from build123d import *

# Parameters (mm, degrees)
AXLE_BASE_SKETCH_R        = 15.5
AXLE_DEPTH                = 92
GUARD_BASE_R              = 25
GUARD_DEPTH               = 5
INNER_AXLE_HOLE_BASE_R    = 10
INNER_AXLE_HOLE_DEPTH     = 104.242433137
COUPLING_TOOTH_HOLE_DEPTH = 4


with BuildPart() as part:
    # Axle base sketch → Axle (new body)
    with BuildSketch(Plane.XY):
        Circle(AXLE_BASE_SKETCH_R)
    extrude(amount=AXLE_DEPTH)

    # Guard base → Guard (add)
    with BuildSketch(Plane(origin=(0, 0, 0), x_dir=(-1, 0, 0), z_dir=(0, 0, -1))):
        Circle(GUARD_BASE_R)
    extrude(amount=GUARD_DEPTH)

    # Inner axle hole base → Inner axle hole (cut, through all)
    with BuildSketch(Plane.XY.offset(92)):
        Circle(INNER_AXLE_HOLE_BASE_R)
    extrude(amount=-INNER_AXLE_HOLE_DEPTH, mode=Mode.SUBTRACT)

    # Coupling tooth base → Coupling tooth hole (cut, symmetric)
    with BuildSketch(Plane(origin=(0, 0, 0), x_dir=(1, 0, 0), z_dir=(0, 1, 0))):
        Polygon((12.5, -89.5), (10, -92), (15.5, -92), (15.5, -79), (12.5, -79), (11.5, -80), (11.5, -82), (12.5, -83), align=None)
    coupling_tooth_hole = extrude(amount=COUPLING_TOOTH_HOLE_DEPTH, both=True, mode=Mode.SUBTRACT)

    # Coupling teeth: Coupling tooth hole across plane
    add(coupling_tooth_hole.mirror(Plane(origin=(0, 0, 0), x_dir=(0, 0, 1), z_dir=(1, 0, 0))), mode=Mode.SUBTRACT)


solid = part.part
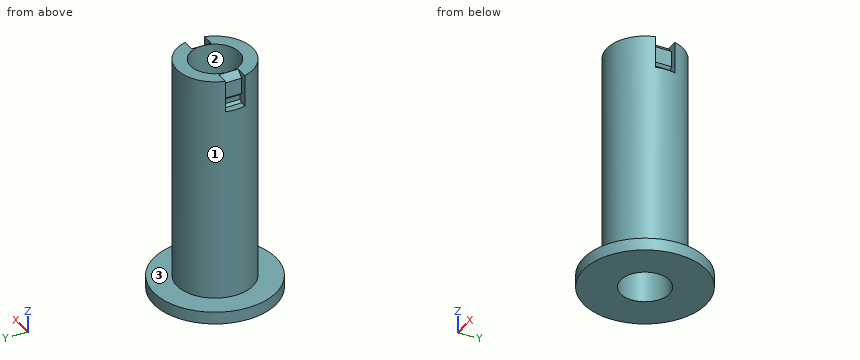
Could you check a few things on this model? Use its own coordinates, in mm. Face numbers are marked on the shaded views. Give positions to 0.01 mm unless a question says otherwise; leave off trailing zeros. Order: outer loops, then holes, each group sorted by start corner. A loop starts at its lowest first (then second) coordinate and runs counter-clockwise, first axis right, second up.
1. Suppose I cut it at D-D (y = -14.5). List the corners of the cut face in (x, z) for me.
2. Will these pins go through, and if not, where does the flat tip stop? P1, Ø12, axis at x = 15.5, z = 22, coming from the +Y side; P2, Ø5, axis at x = -18.5, y = -18.5, coming from the +Z side; P3, Ø12, axis at x = 15, z = 65.5, coming from the -Y side; P4, Ø12, axis at x = -9, y = -18.5, coming from the +Z side.
3. Suppose I cut it at C-C (z = 70.5). List the corners of the cut face in (x, y) for me.
4. Suppose I cut it at B-B (y = -6.5). List the corners of the cut face in (x, z) for me, plus the area to 3 significant figures.
5. I need wall thicknesses on L1, parallel to Y at x = 0, z = 22; L2, parallel to Z at x = -11, y = -15.5; L3, parallel to Y at x = 8.5, z = 10.5. Which ranges of each line are inside material? Lowest first, please.
6. Suppose I cut it at A-A (x = 0). List the corners of the cut face in (y, z) for me, plus the area to 3 significant figures.
7. We'd pull the mould along Y, two halves only. Please class the marked faces 1, 2 and 3: pulls with the +Y half, pulls with the -Y half, needs draft (parallel to the pull), parting line crosses it, or undercut.
Solved:
1. outline: (-20.37, -5) - (20.37, -5) - (20.37, 0) - (5.48, 0) - (5.48, 92) - (-5.48, 92) - (-5.48, 0) - (-20.37, 0) - close
2. P1: stops at y = 12.25
2. P2: stops at z = 0
2. P3: stops at y = -12.62
2. P4: stops at z = 92
3. outline: circle Ø31 at (0, 0); hole circle Ø20 at (0, 0)
4. outline: (-24.14, -5) - (-7.6, -5) - (-7.6, 92) - (-14.07, 92) - (-14.07, 0) - (-24.14, 0) - close; (7.6, -5) - (24.14, -5) - (24.14, 0) - (14.07, 0) - (14.07, 92) - (7.6, 92) - close
4. area: 1,360 mm2
5. L1: y = -15.5 to -10, 10 to 15.5
5. L2: z = -5 to 0
5. L3: y = -12.96 to -5.27, 5.27 to 12.96
6. outline: (-25, -5) - (-10, -5) - (-10, 92) - (-15.5, 92) - (-15.5, 0) - (-25, 0) - close; (10, -5) - (25, -5) - (25, 0) - (15.5, 0) - (15.5, 92) - (10, 92) - close
6. area: 1,160 mm2
7. face 1: parting line crosses it
7. face 2: undercut
7. face 3: needs draft
